Work out the finished part from the listing and answer in its coordinate system (mm). Face numbers are marked on the shaded views. A direction names the side the tool comes from. Give positions to 0.01 mm unless a question says otherwise; leave off trailing zeros. Loops run counter-clockwise (first coordinate to the right, second up) from the corner with the lowest first, then second, coordinate; pieces in that order, holes last. Notation, with made-up numbers: (18.25, 10) - (45.25, 10) arc R8 cw to (45.25, 24) - close; hole circle Ø9 at (75, 71.25). An arc over 180 degrees is marked (long way). One line per question, with ' | ' between items.
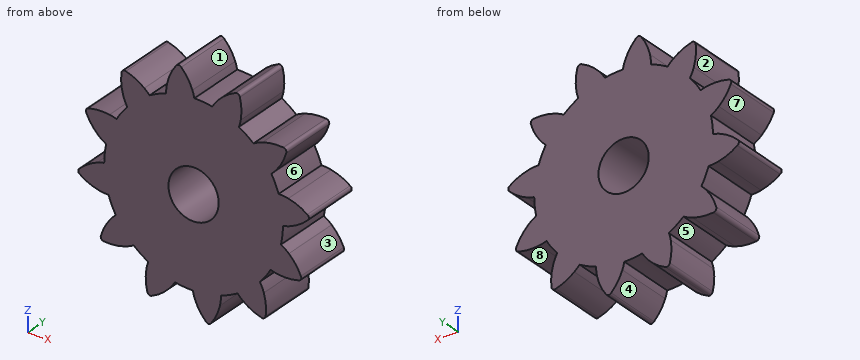
from build123d import *

# Parameters (mm, degrees)
F0_R     = 7.5523457901
F1_DEPTH = 18
F2_COUNT = 12


with BuildPart() as f1:
    # F0 (on Front) → F1 (new body)
    with BuildSketch(Plane.XZ):
        with BuildLine():
            ThreePointArc((-8.2701024402, 25.55566211), (-15.8010660029, -21.7212516541), (26.8605, 0))
            ThreePointArc((26.8605, 0), (19.0736413542, 18.9125002509), (0.2278858833, 26.8595332847))
            ThreePointArc((0.2278858833, 26.8595332847), (-4.0736140952, 26.5498046782), (-8.2701024402, 25.55566211))
        make_face()
        Circle(F0_R, mode=Mode.SUBTRACT)
        with BuildLine():
            ThreePointArc((-8.2701024402, 25.55566211), (-4.0736140952, 26.5498046782), (0.2278858833, 26.8595332847))
            ThreePointArc((0.2278858833, 26.8595332847), (-0.0259637004, 27.9265875849), (-0.3583119198, 28.971857479))
            ThreePointArc((-0.3583119198, 28.971857479), (-1.7585942686, 31.8051493547), (-3.7177759967, 34.2850567048))
            ThreePointArc((-3.7177759967, 34.2850567048), (-4.5350574201, 34.6527650776), (-5.2973513139, 34.1815258688))
            ThreePointArc((-5.2973513139, 34.1815258688), (-6.9160791073, 31.467109939), (-7.9345630465, 28.475283745))
            ThreePointArc((-7.9345630465, 28.475283745), (-8.1751413026, 27.023840498), (-8.2701024402, 25.55566211))
        make_face()
    extrude(amount=F1_DEPTH)

    # F2: F1 ×12 about axis
    f2_axis = Axis((0, 0, 0), (0, 1, 0))


with BuildPart() as f1_1:
    add(f1.part)
    for i in range(1, F2_COUNT):
        add(f1.part.rotate(f2_axis, i * 360 / F2_COUNT))


solid = f1_1.part
1. Determine the mould class of the marked faces 5, 6, 7 and 8 for opening direction X: +X half, -X half, draft (parallel to the pull), parting line (faces both ways), or undercut.
Evaluation:
face 5: undercut | face 6: +X half | face 7: -X half | face 8: undercut
2. Which of the six approach directions +Z, -Z, +X, -X, +Y, -Y give full straight-line access (tool end or side, diameter ignored) to the marked faces 1, 2, 3 and 4?
Evaluation:
face 1: +Z, +Y, -Y | face 2: -X, +Y, -Y | face 3: +X, +Y, -Y | face 4: -Z, +Y, -Y
3. Find section A-A on x = -10. Write down the section's boundary in (y, z), then the cut area to 3 significant figures.
Evaluation:
outline: (-18, -30.89) - (0, -30.89) - (0, 24.93) - (-18, 24.93) - close | area: 1,000 mm2
4. Consider L1, parallel to X at y = -6, z = 30.5; L2, parallel to Z at x = 4, y = -13; L3, parallel to Z at x = 6, y = -2.75. Determine where each line is inside the solid, lowest interval first.
Evaluation:
L1: -7.32 to -1.02, 9.45 to 14.15 | L2: -34.53 to -6.41, 6.41 to 26.56 | L3: -33.16 to -4.59, 4.59 to 26.88
5. Flat-ended cylindrical pins translate along their axes: pin 1 (5 mm diameter, centred on y = -9, z = 25.5, fed in from +X); pin 2 (3 mm diameter, centred on y = -5, z = 10.5, fed in from -X); pin 3 (6 mm diameter, centred on y = -11.5, z = 14, fed in from -X); pin 4 (13.5 mm diameter, centred on x = 0, z = 0, fed in from +Y). Find the tip coordinate at first contact, or state that the pin passes through.
Evaluation:
pin 1: x = 14.39 | pin 2: x = -32.02 | pin 3: x = -32.38 | pin 4: through
